Autodesk Inventor part; units mm, degrees
ref_plane "YZ Plane" through (0, 0, 0) normal (1, 0, 0) x (0, 1, 0)
ref_plane "XZ Plane" through (0, 0, 0) normal (0, 1, 0) x (-1, 0, 0)
ref_plane "XY Plane" through (0, 0, 0) normal (0, 0, 1) x (1, 0, 0)
sketch "Sketch1" plane through (0, 0, 0) normal (0, 1, 0) x (-1, 0, 0)
  circle A0 centre (0, 0) radius 25
  dimension "d0" = 50
extrude "Extrusion1" add sketch "Sketch1" along normal blind 5
sketch "Sketch2" plane through (0, 5, 0) normal (0, 1, 0) x (1, 0, 0)
  circle A0 centre (0, 0) radius 7.5
  dimension "d3" = 15
extrude "Extrusion2" cut sketch "Sketch2" against normal through all
sketch "Sketch3" plane through (0, 5, 0) normal (0, 1, 0) x (1, 0, 0)
  circle A0 centre (0, 0) radius 20 construction
sketch "Sketch4" plane through (0, 5, 0) normal (0, 1, 0) x (1, 0, 0)
  circle A0 centre (0, -20) radius 2.5
  point P0 (0, 0)
  dimension "d8" = 5
extrude "Extrusion3" cut sketch "Sketch4" against normal through all
sketch "Sketch5" plane through (0, 5, 0) normal (0, 1, 0) x (1, 0, 0)
  line L0 (0, 0) -> (-12.8558, 15.3209)
  line L1 (0, 0) -> (0, -27.4763)
  arc A0 (-10.0367, 16.3469) -> (-15.6748, 14.2948) centre (-12.8558, 15.3209) ccw
  arc A1 (-2.8191, -21.0261) -> (2.8191, -18.9739) centre (0, -20) ccw
  line L2 (-10.0367, 16.3469) -> (2.8191, -18.9739)
  line L3 (-2.8191, -21.0261) -> (-15.6748, 14.2948)
  circle A2 centre (0, 0) radius 3
  dimension "d11" = 140
  dimension "d14" = 20
  dimension "d15" = 3
  dimension "d17" = 3
  dimension "d18" = 6
properties part number "test wysiegu sprezyny"
Geometry: final body of the model. Coordinates: model frame, mm. Round coordinates to 2 decimals unless told otherwise and drop trailing zeros. Loops run counter-clockwise (first coordinate to the right, second up) from the corner with the lowest first, then second, coordinate; pieces in that order, holes last. Notation, with made-up numbers: (-4.5, -5) -> (23.5, -5) arc R22 ccw to (23.5, 12) -> close; hole circle Ø10 at (29.25, -12). An arc over 180 degrees is marked (long way). Use one line per item in the form item = value. Start each with the question number.
1) Section C-C on y = 3.4. Output: boundary loops of the cut face in (x, z), then the cut area to 3 significant figures.
2) Line query: L1, parallel to Z at x = 0, y = 2.4; L2, parallel to X at y = 4.45, z = 20.5; L3, parallel to Z at x = -6, y = 4.15. Output: solid intervals per line, ascending.
3) Draft query along X for faces 1 (the cylindrical face through (1.34, 2.54, 17.89)), 2 (the cylindrical face through (-7.493, 2.535, -0.33)), 3 (the flat face through (-5, 0, 6)), 4 (the cylindrical face through (-23.846, 2.465, -7.509)). Return one class per face: released by +X, released by -X, zero draft, split by the parting line, or undercut.
4) Section B-B on x = -0.5. Output: boundary loops of the cut face in (y, z) (3 decimals), then the cut area to 3 significant figures.
5) Section A-A on z = -4. Output: boundary loops of the cut face in (x, y).
6) First-contact query: P1, Ø2, axis at y = 0.5, z = 17, coming from the +X side; P2, Ø1, axis at y = 1, z = 10.5, coming from the +X side; P3, Ø1, axis at x = 20, y = 4, coming from the +Z side. Flat tips, straight axial feed; report the tip coordinate or a pass-through.
7) Section D-D on z = 4.5. Output: boundary loops of the cut face in (x, y).
Response:
q1.outline = circle Ø50 at (0, 0); hole circle Ø15 at (0, 0); hole circle Ø5 at (0, 20)
q1.area = 1,770 mm^2
q2.L1 = -25 to -7.5, 7.5 to 17.5, 22.5 to 25
q2.L2 = -14.31 to -2.45, 2.45 to 14.31
q2.L3 = -24.27 to -4.5, 4.5 to 24.27
q3.face_1 = undercut
q3.face_2 = undercut
q3.face_3 = zero draft
q3.face_4 = split by the parting line
q4.outline = (0, -24.995) -> (5, -24.995) -> (5, -7.483) -> (0, -7.483) -> close; (0, 7.483) -> (5, 7.483) -> (5, 17.551) -> (0, 17.551) -> close; (0, 22.449) -> (5, 22.449) -> (5, 24.995) -> (0, 24.995) -> close
q4.area = 151 mm^2
q5.outline = (-24.68, 0) -> (-6.34, 0) -> (-6.34, 5) -> (-24.68, 5) -> close; (6.34, 0) -> (24.68, 0) -> (24.68, 5) -> (6.34, 5) -> close
q6.P1 = 19.21
q6.P2 = 22.91
q6.P3 = 15.64
q7.outline = (-24.59, 0) -> (-6, 0) -> (-6, 5) -> (-24.59, 5) -> close; (6, 0) -> (24.59, 0) -> (24.59, 5) -> (6, 5) -> close
